Here's how the part is built. I have some questions about the finished solid (model axes, mm). Face numbers are marked on the shaded views. A direction names the side the tool comes from. Round coordinates to 2 decimals unless told otherwise and drop trailing zeros. Write each loop counter-clockwise with the first axis right and the second up, starting at its lowest first coordinate (ties: lowest second). Pieces come first, ordered by that corner, then holes. Notation, with made-up numbers: (-7, 83.25) -> (17, 83.25) arc R20 ccw to (17, 93.25) -> close; hole circle Ø3 at (12.25, 31.25). An arc over 180 degrees is marked (long way). Answer as CSV lines item,"result".
```python
from build123d import *

# Parameters (mm, degrees)
SKETCH3_R                = 4.242640687
BOSS_EXTRUDE1_DEPTH      = 10
FILLET1_R                = 1.5
BOSS_EXTRUDE2_DEPTH      = 5
FILLET2_R                = 5
SKETCH5_W                = 13
SKETCH5_H                = 13
BOSS_EXTRUDE3_DEPTH      = 45
CUT_EXTRUDE4_REACH       = 48.503
SKETCH6_W                = 13
SKETCH6_H                = 4.7
SKETCH6_H_2              = 7.2
BOSS_EXTRUDE4_DEPTH      = 2
BOSS_EXTRUDE4_DEPTH_BACK = 5.5
SKETCH9_R                = 3
BOSS_EXTRUDE5_DEPTH      = 2
BOSS_EXTRUDE5_DEPTH_BACK = 5.5
SKETCH10_R               = 3
BOSS_EXTRUDE6_DEPTH      = 2
BOSS_EXTRUDE6_DEPTH_BACK = 5.5
SKETCH12_R               = 3
BOSS_EXTRUDE7_DEPTH      = 2
BOSS_EXTRUDE7_DEPTH_BACK = 5.5
SKETCH14_R               = 3
FILLET4_R                = 2
FILLET8_R                = 2


with BuildPart() as part:
    # Sketch1 → Revolve1 (revolve)
    with BuildSketch(Plane(origin=(0, 0, 0), x_dir=(1, 0, 0), z_dir=(0, 1, 0))):
        with BuildLine():
            Line((-9.5, 0), (8.5, 0))
            Line((8.5, 0), (8.5, 4.242640687))
            ThreePointArc((8.5, 4.242640687), (-2.179449472, 9.246621004), (-9.5, 0))
        make_face()
    revolve(axis=Axis((-9.5, 0, 0), (1, 0, 0)))

    # Sketch3 → Boss-Extrude1 (add)
    with BuildSketch(Plane(origin=(8.5, 0, 0), x_dir=(0, 0, -1), z_dir=(1, 0, 0))):
        Circle(SKETCH3_R)
    extrude(amount=BOSS_EXTRUDE1_DEPTH)

    # Fillet1
    fillet1_edges = [part.edges().sort_by_distance(p)[0] for p in [
        (8.5, 0, 4.242640687),
    ]]
    fillet(fillet1_edges, radius=FILLET1_R)

    # Sketch4 → Boss-Extrude2 (add)
    with BuildSketch(Plane(origin=(18.5, 0, 0), x_dir=(0, 0, -1), z_dir=(1, 0, 0))):
        with BuildLine():
            Line((19.5, -10), (-19.5, -10))
            ThreePointArc((-19.5, -10), (-21.621320344, -9.121320344), (-22.5, -7))
            Line((-22.5, -7), (-22.5, 7))
            ThreePointArc((-22.5, 7), (-21.621320344, 9.121320344), (-19.5, 10))
            Line((-19.5, 10), (19.5, 10))
            ThreePointArc((19.5, 10), (21.621320344, 9.121320344), (22.5, 7))
            Line((22.5, 7), (22.5, -7))
            ThreePointArc((22.5, -7), (21.621320344, -9.121320344), (19.5, -10))
        make_face()
    extrude(amount=BOSS_EXTRUDE2_DEPTH)

    # Fillet2
    fillet2_edges = [part.edges().sort_by_distance(p)[0] for p in [
        (18.5, 0, 4.242640687),
    ]]
    fillet(fillet2_edges, radius=FILLET2_R)

    # Sketch5 → Boss-Extrude3 (add, through all)
    with BuildSketch(Plane.XY.offset(22.5)):
        with Locations((30, 1.5)):
            Rectangle(SKETCH5_W, SKETCH5_H)
    extrude(amount=-BOSS_EXTRUDE3_DEPTH)

    # Sketch6 → Cut-Extrude4 (cut, up to next)
    with BuildSketch(Plane(origin=(0, 8, 0), x_dir=(1, 0, 0), z_dir=(0, 1, 0)), mode=Mode.PRIVATE) as cut_extrude4_sk1:
        with Locations((30, -20.15)):
            Rectangle(SKETCH6_W, SKETCH6_H)
    cut_extrude4_tool1 = extrude(cut_extrude4_sk1.sketch, amount=-CUT_EXTRUDE4_REACH, mode=Mode.PRIVATE) & part.part
    # Sketch6 → Cut-Extrude4 (cut, up to next)
    with BuildSketch(Plane(origin=(0, 8, 0), x_dir=(1, 0, 0), z_dir=(0, 1, 0)), mode=Mode.PRIVATE) as cut_extrude4_sk2:
        with Locations((30, -10.7)):
            Rectangle(SKETCH6_W, SKETCH6_H_2)
    cut_extrude4_tool2 = extrude(cut_extrude4_sk2.sketch, amount=-CUT_EXTRUDE4_REACH, mode=Mode.PRIVATE) & part.part
    # Sketch6 → Cut-Extrude4 (cut, up to next)
    with BuildSketch(Plane(origin=(0, 8, 0), x_dir=(1, 0, 0), z_dir=(0, 1, 0)), mode=Mode.PRIVATE) as cut_extrude4_sk3:
        with Locations((30, 0)):
            Rectangle(SKETCH6_W, SKETCH6_H_2)
    cut_extrude4_tool3 = extrude(cut_extrude4_sk3.sketch, amount=-CUT_EXTRUDE4_REACH, mode=Mode.PRIVATE) & part.part
    # Sketch6 → Cut-Extrude4 (cut, up to next)
    with BuildSketch(Plane(origin=(0, 8, 0), x_dir=(1, 0, 0), z_dir=(0, 1, 0)), mode=Mode.PRIVATE) as cut_extrude4_sk4:
        with Locations((30, 10.7)):
            Rectangle(SKETCH6_W, SKETCH6_H_2)
    cut_extrude4_tool4 = extrude(cut_extrude4_sk4.sketch, amount=-CUT_EXTRUDE4_REACH, mode=Mode.PRIVATE) & part.part
    # Sketch6 → Cut-Extrude4 (cut, up to next)
    with BuildSketch(Plane(origin=(0, 8, 0), x_dir=(1, 0, 0), z_dir=(0, 1, 0)), mode=Mode.PRIVATE) as cut_extrude4_sk5:
        with Locations((30, 20.15)):
            Rectangle(SKETCH6_W, SKETCH6_H)
    cut_extrude4_tool5 = extrude(cut_extrude4_sk5.sketch, amount=-CUT_EXTRUDE4_REACH, mode=Mode.PRIVATE) & part.part
    add(cut_extrude4_tool1.solids().sort_by_distance((30, 8, 20.15))[0], mode=Mode.SUBTRACT)
    add(cut_extrude4_tool2.solids().sort_by_distance((30, 8, 10.7))[0], mode=Mode.SUBTRACT)
    add(cut_extrude4_tool3.solids().sort_by_distance((30, 8, 0))[0], mode=Mode.SUBTRACT)
    add(cut_extrude4_tool4.solids().sort_by_distance((30, 8, -10.7))[0], mode=Mode.SUBTRACT)
    add(cut_extrude4_tool5.solids().sort_by_distance((30, 8, -20.15))[0], mode=Mode.SUBTRACT)

    # Sketch9 → Boss-Extrude4 (add, two sides: drawn at the far end of the back side and taken through both)
    with BuildSketch(Plane.XY.offset(17.8).offset(-BOSS_EXTRUDE4_DEPTH_BACK)):
        with Locations((31.5, 1.5)):
            Circle(SKETCH9_R)
    extrude(amount=BOSS_EXTRUDE4_DEPTH + BOSS_EXTRUDE4_DEPTH_BACK)

    # Sketch10 → Boss-Extrude5 (add, two sides: drawn at the far end of the back side and taken through both)
    with BuildSketch(Plane.XY.offset(7.1).offset(-BOSS_EXTRUDE5_DEPTH_BACK)):
        with Locations((31.5, 1.5)):
            Circle(SKETCH10_R)
    extrude(amount=BOSS_EXTRUDE5_DEPTH + BOSS_EXTRUDE5_DEPTH_BACK)

    # Sketch12 → Boss-Extrude6 (add, two sides: drawn at the far end of the back side and taken through both)
    with BuildSketch(Plane.XY.offset(-3.6).offset(-BOSS_EXTRUDE6_DEPTH_BACK)):
        with Locations((31.5, 1.5)):
            Circle(SKETCH12_R)
    extrude(amount=BOSS_EXTRUDE6_DEPTH + BOSS_EXTRUDE6_DEPTH_BACK)

    # Sketch14 → Boss-Extrude7 (add, two sides: drawn at the far end of the back side and taken through both)
    with BuildSketch(Plane.XY.offset(-14.3).offset(-BOSS_EXTRUDE7_DEPTH_BACK)):
        with Locations((31.5, 1.5)):
            Circle(SKETCH14_R)
    extrude(amount=BOSS_EXTRUDE7_DEPTH + BOSS_EXTRUDE7_DEPTH_BACK)

    # Fillet4
    fillet4_edges = [part.edges().sort_by_distance(p)[0] for p in [
        (23.5, -5, -16.05),
        (23.5, -5, -5.35),
        (23.5, -5, 5.35),
        (23.5, -5, 16.05),
        (23.5, 8, -16.05),
        (23.5, 8, -5.35),
        (23.5, 8, 5.35),
        (23.5, 8, 16.05),
    ]]
    fillet(fillet4_edges, radius=FILLET4_R - 0.0001)  # a hair under: the kernel refuses the full size

    # Fillet8
    fillet8_edges = [part.edges().sort_by_distance(p)[0] for p in [
        (18.5, -9.121320344, 21.621320344),
        (18.5, -10, 0),
        (18.5, -9.121320344, -21.621320344),
        (18.5, 0, -22.5),
        (18.5, 9.121320344, -21.621320344),
        (18.5, 10, 0),
        (18.5, 9.121320344, 21.621320344),
        (18.5, 0, 22.5),
    ]]
    fillet(fillet8_edges, radius=FILLET8_R)


solid = part.part
```
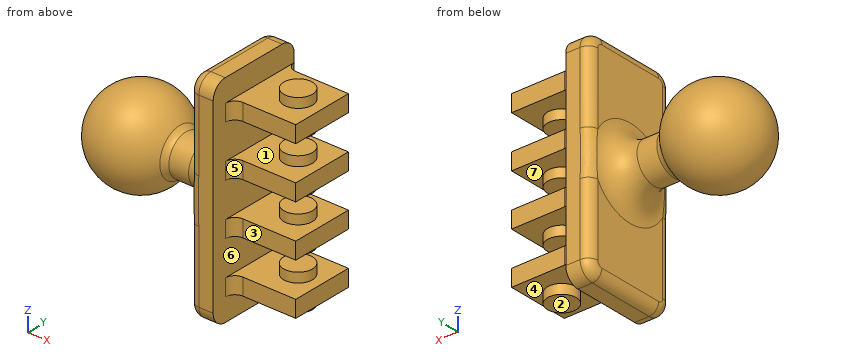
1. For pin 1 Ø3 at (x, y) = (32.5, 1.5) entering from -Z; pin 2 Ø3 at (x, z) = (28.5, -16) entering from -Y; pin 3 Ø4 at (x, y) = (1, 7.5) entering from -Z; pin 4 Ø8 at (x, z) = (26, 0.5) entering from -Y, each with a flat end and sliding along its axis, tell me the tip position at first contact or that it passes through.
Numbers:
pin 1,"stops at z = -19.8"
pin 2,"stops at y = -5"
pin 3,"stops at z = -7.7"
pin 4,"stops at y = -10"
2. Suppose I cut it at A-A on z = 18.5. Please give me the cut outline in (x, y), and give its area (3 significant figures).
Numbers:
outline,"(18.5, -8) arc R2 ccw to (20.5, -10) -> (23.5, -10) -> (23.5, 10) -> (20.5, 10) arc R2 ccw to (18.5, 8) -> close; circle Ø6 at (31.5, 1.5)"
area,"127 mm^2"
3. If we mould it in two halves opening along Z, with no side actions, what happens to the marked faces 4, 5, 6 and 7? For each: released by +Z, released by -Z, zero draft, split by the parting line, or undercut.
Numbers:
face 4,"released by -Z"
face 5,"zero draft"
face 6,"undercut"
face 7,"undercut"
4. Suppose I cut it at B-B on x = 31.5. Count the separate pieces of the cut face and the enclosed holes in it, and give its area (3 significant figures).
Numbers:
separate pieces,"4"
enclosed holes,"0"
area,"278 mm^2"
5. If I drill on line 1 (Z direction, x = 27, y = -1); line 2 (X direction, y = -8, z = -18.5); line 3 (X direction, y = 3.5, z = -16.5), over which ranges is the centre line in solid material (lowest first)?
Numbers:
line 1,"z = -17.8 to -14.3, -7.1 to -3.6, 3.6 to 7.1, 14.3 to 17.8"
line 2,"x = 18.5 to 23.5"
line 3,"x = 18.5 to 36.5"
6. Suppose I cut it at D-D on x = 16.5. Please give me the cut outline in (y, z), and give its area (3 significant figures).
Numbers:
outline,"circle Ø10.49 at (0, 0)"
area,"86.3 mm^2"
7. On a 3-axis mill with a long thin cutter (end or side, diameter ignored), from which of +Z, -Z, +X, -X, +Y, -Y can I reach the whole of each face in a straight line? I mean the marked faces 1, 2 and 3. Say none if no direction works.
Numbers:
face 1,"none"
face 2,"-Z, +X, +Y, -Y"
face 3,"+Z, -Z, +X, -Y"
8. Suppose I cut it at C-C on x = 7.5. Please give me the cut outline in (y, z), and give its area (3 significant figures).
Numbers:
outline,"circle Ø11.66 at (0, 0)"
area,"107 mm^2"
